Verification items for the finished model (mm, model axes). A direction names the side the tool comes from. Round coordinates to 2 decimals unless told otherwise and drop trailing zeros. Loops run counter-clockwise (first coordinate to the right, second up) from the corner with the lowest first, then second, coordinate; pieces in that order, holes last.
from build123d import *

# Parameters (mm, degrees)
F1_DEPTH = 25.4
F2_R     = 63.5
F3_DEPTH = 152.4
F6_R     = 57.15
F7_DEPTH = 228.6
F8_R     = 69.85
F8_R_2   = 57.15
F9_DEPTH = 6.35


with BuildPart() as f1:
    # F0 (on Front) → F1 (new body)
    with BuildSketch(Plane.XZ):
        with BuildLine():
            ThreePointArc((99.175375, -22.063657), (100.992025, -11.098241), (101.6, 0))
            ThreePointArc((101.6, 0), (100.992025, 11.098241), (99.175375, 22.063657))
            ThreePointArc((99.175375, 22.063657), (87.988181, 50.8), (68.695375, 74.856566))
            ThreePointArc((68.695375, 74.856566), (50.8, 87.988181), (30.48, 96.920223))
            ThreePointArc((30.48, 96.920223), (0, 101.6), (-30.48, 96.920223))
            ThreePointArc((-30.48, 96.920223), (-50.8, 87.988181), (-68.695375, 74.856566))
            ThreePointArc((-68.695375, 74.856566), (-87.988181, 50.8), (-99.175375, 22.063657))
            ThreePointArc((-99.175375, 22.063657), (-101.6, 0), (-99.175375, -22.063657))
            ThreePointArc((-99.175375, -22.063657), (-87.988181, -50.8), (-68.695375, -74.856566))
            ThreePointArc((-68.695375, -74.856566), (-50.8, -87.988181), (-30.48, -96.920223))
            ThreePointArc((-30.48, -96.920223), (0, -101.6), (30.48, -96.920223))
            ThreePointArc((30.48, -96.920223), (50.8, -87.988181), (68.695375, -74.856566))
            ThreePointArc((68.695375, -74.856566), (87.988181, -50.8), (99.175375, -22.063657))
        make_face()
        with BuildLine():
            ThreePointArc((-30.48, 96.920223), (0, 101.6), (30.48, 96.920223))
            Line((30.48, 96.920223), (30.48, 102.87))
            ThreePointArc((30.48, 102.87), (24.900384, 116.340384), (11.43, 121.92))
            Line((11.43, 121.92), (-11.43, 121.92))
            ThreePointArc((-11.43, 121.92), (-24.900384, 116.340384), (-30.48, 102.87))
            Line((-30.48, 102.87), (-30.48, 96.920223))
        make_face()
        with BuildLine():
            ThreePointArc((68.695375, 74.856566), (87.988181, 50.8), (99.175375, 22.063657))
            Line((99.175375, 22.063657), (104.328033, 25.038546))
            ThreePointArc((104.328033, 25.038546), (113.20392, 36.605827), (111.300817, 51.06133))
            Line((111.300817, 51.06133), (99.870817, 70.85867))
            ThreePointArc((99.870817, 70.85867), (88.303536, 79.734557), (73.848033, 77.831454))
            Line((73.848033, 77.831454), (68.695375, 74.856566))
        make_face()
        with BuildLine():
            Line((104.328033, -25.038546), (99.175375, -22.063657))
            ThreePointArc((99.175375, -22.063657), (87.988181, -50.8), (68.695375, -74.856566))
            Line((68.695375, -74.856566), (73.848033, -77.831454))
            ThreePointArc((73.848033, -77.831454), (88.303536, -79.734557), (99.870817, -70.85867))
            Line((99.870817, -70.85867), (111.300817, -51.06133))
            ThreePointArc((111.300817, -51.06133), (113.20392, -36.605827), (104.328033, -25.038546))
        make_face()
        with BuildLine():
            Line((30.48, -102.87), (30.48, -96.920223))
            ThreePointArc((30.48, -96.920223), (0, -101.6), (-30.48, -96.920223))
            Line((-30.48, -96.920223), (-30.48, -102.87))
            ThreePointArc((-30.48, -102.87), (-24.900384, -116.340384), (-11.43, -121.92))
            Line((-11.43, -121.92), (11.43, -121.92))
            ThreePointArc((11.43, -121.92), (24.900384, -116.340384), (30.48, -102.87))
        make_face()
        with BuildLine():
            Line((-73.848033, -77.831454), (-68.695375, -74.856566))
            ThreePointArc((-68.695375, -74.856566), (-87.988181, -50.8), (-99.175375, -22.063657))
            Line((-99.175375, -22.063657), (-104.328033, -25.038546))
            ThreePointArc((-104.328033, -25.038546), (-113.20392, -36.605827), (-111.300817, -51.06133))
            Line((-111.300817, -51.06133), (-99.870817, -70.85867))
            ThreePointArc((-99.870817, -70.85867), (-88.303536, -79.734557), (-73.848033, -77.831454))
        make_face()
        with BuildLine():
            ThreePointArc((-99.175375, 22.063657), (-87.988181, 50.8), (-68.695375, 74.856566))
            Line((-68.695375, 74.856566), (-73.848033, 77.831454))
            ThreePointArc((-73.848033, 77.831454), (-88.303536, 79.734557), (-99.870817, 70.85867))
            Line((-99.870817, 70.85867), (-111.300817, 51.06133))
            ThreePointArc((-111.300817, 51.06133), (-113.20392, 36.605827), (-104.328033, 25.038546))
            Line((-104.328033, 25.038546), (-99.175375, 22.063657))
        make_face()
    extrude(amount=F1_DEPTH)

    # F2 (on face) → F3 (join)
    with BuildSketch(Plane(origin=(0, 0, 0), x_dir=(-1, 0, 0), z_dir=(0, 1, 0))):
        Circle(F2_R)
    extrude(amount=F3_DEPTH)

    # F5: F1 across plane


with BuildPart() as f1_1:
    add(f1.part)
    add(f1.part.mirror(Plane(origin=(0, 76.2, 0), x_dir=(1, 0, 0), z_dir=(0, 1, 0))))

    # F6 (on face) → F7 (cut)
    with BuildSketch(Plane.XZ.offset(25.4)):
        Circle(F6_R)
    extrude(amount=-F7_DEPTH, mode=Mode.SUBTRACT)

    # F8 (on face) → F9 (cut)
    with BuildSketch(Plane.XZ.offset(25.4)):
        Circle(F8_R)
        Circle(F8_R_2, mode=Mode.SUBTRACT)
    extrude(amount=-F9_DEPTH, mode=Mode.SUBTRACT)

    # F10: F1 across plane


with BuildPart() as f1_2:
    add(f1_1.part)
    add(f1_1.part.mirror(Plane(origin=(0, 76.2, 0), x_dir=(1, 0, 0), z_dir=(0, 1, 0))), mode=Mode.INTERSECT)


solid = f1_2.part
1. Section check B-B (z = -33). Enter the section's corners in (x, y).
2. Scan lines: L1, parallel to Y at x = 59, z = -36; L2, parallel to Y at x = -21.5, z = 69; L3, parallel to Z at x = 0, y = 80.5. Record each from-to range of solid material in increasing order.
3. Section check A-A (x = 0). Enter the section's corners in (y, z).
4. Release check for a two-part mould opening along Z. For faces 6 (the face through (-50.53, -12.522, 88.143)), 7 (the face through (-113.257, 164.922, 36.808)), 8 (the face through (-25.05, -12.52, -116.19)) record: released by +Z, released by -Z, zero draft, split by the parting line, or undercut.
5. Gauge pin test, flat ends, axial feed: P1, Ø2, axis at x = -47, y = 14, coming from the -Z side (3 decimals); P2, Ø3, axis at y = 161, z = 101, coming from the -X side; P3, Ø3, axis at x = 42, y = 71.5, coming from the -Z side. Record the tip position at first contact, or that the pin passes through.
6. Tool access check on faces 1 (the face through (-55.431, -22.269, -42.503)), 2 (the face through (105.506, -12.522, -61.099)), 3 (the face through (-30.48, -13, -100)), 4 (the face through (-57.095, 74.866, 2.513)), 5 (the face through (50.53, 164.922, -88.143)). Record the directions out of +Z, -Z, +X, -X, +Y, -Y that give a thin tool (end or side, any length) a straight path to the whole face; none if there is none.
7. Section check C-C (y = 36.5). Enter the section's corners in (x, z), then the cut area to 3 significant figures.
Taken from the geometry:
1. outline: (-111.83, -25.4) - (-61.56, -25.4) - (-61.56, -19.05) - (-46.66, -19.05) - (-46.66, 171.45) - (-61.56, 171.45) - (-61.56, 177.8) - (-111.83, 177.8) - (-111.83, 152.4) - (-54.25, 152.4) - (-54.25, 0) - (-111.83, 0) - close; (46.66, -19.05) - (61.56, -19.05) - (61.56, -25.4) - (111.83, -25.4) - (111.83, 0) - (54.25, 0) - (54.25, 152.4) - (111.83, 152.4) - (111.83, 177.8) - (61.56, 177.8) - (61.56, 171.45) - (46.66, 171.45) - close
2. L1: y = -19.05 to 0, 152.4 to 171.45
2. L2: y = -25.4 to 0, 152.4 to 177.8
2. L3: z = -63.5 to -57.15, 57.15 to 63.5
3. outline: (-25.4, -121.92) - (0, -121.92) - (0, -63.5) - (152.4, -63.5) - (152.4, -121.92) - (177.8, -121.92) - (177.8, -69.85) - (171.45, -69.85) - (171.45, -57.15) - (-19.05, -57.15) - (-19.05, -69.85) - (-25.4, -69.85) - close; (-25.4, 69.85) - (-19.05, 69.85) - (-19.05, 57.15) - (171.45, 57.15) - (171.45, 69.85) - (177.8, 69.85) - (177.8, 121.92) - (152.4, 121.92) - (152.4, 63.5) - (0, 63.5) - (0, 121.92) - (-25.4, 121.92) - close
4. face 6: released by +Z
4. face 7: undercut
4. face 8: released by -Z
5. P1: stops at z = -43.775
5. P2: stops at x = -30.48
5. P3: stops at z = -48.91
6. face 1: -Y
6. face 2: -Z, +X, +Y, -Y
6. face 3: -Z, -X, +Y, -Y
6. face 4: +Y, -Y
6. face 5: -Z, +Y, -Y
7. outline: circle Ø127 at (0, 0); hole circle Ø114.3 at (0, 0)
7. area: 2,410 mm2
